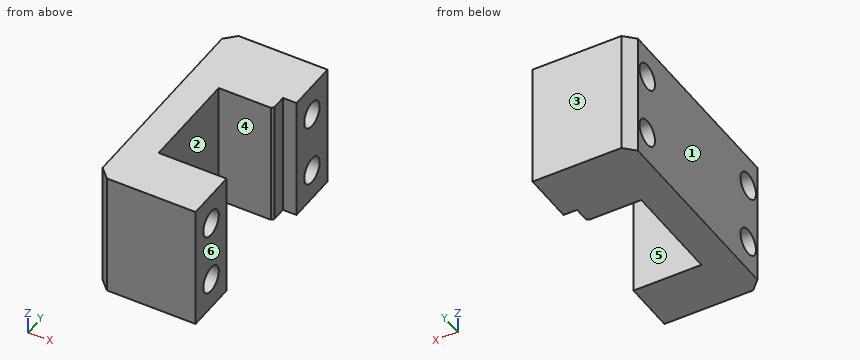
from build123d import *

# Parameters (mm, degrees)
EXTRUDE_1_DEPTH    = 12
CHAMFER_1_SIZE     = 0.2
HOLE_WIZARD_M3_2_D = 2.5
CHAMFER_2_SIZE     = 1


with BuildPart() as part:
    # 草图1 → 凸台-拉伸1 (new body)
    with BuildSketch(Plane.XY):
        Polygon((0, 0), (0, 21.31), (9.5, 21.31), (9.5, 16.31), (8.2, 16.31), (8.2, 14.71), (3, 14.71), (3, 5), (9.5, 5), (9.5, 0), align=None)
    extrude(amount=EXTRUDE_1_DEPTH)

    # 倒角1
    chamfer_1_edges = [part.edges().sort_by_distance(p)[0] for p in [
        (8.2, 14.71, 6),
    ]]
    chamfer(chamfer_1_edges, length=CHAMFER_1_SIZE)

    # M3 螺纹孔2 (through all)
    with Locations(Plane(origin=(0, 2.5, 3), x_dir=(0, 0, -1), z_dir=(-1, 0, 0))):
        with Locations((0, 0), (-6, 0), (-6, -16.31), (0, -16.31)):
            Hole(HOLE_WIZARD_M3_2_D / 2)

    # 倒角2
    chamfer_2_edges = [part.edges().sort_by_distance(p)[0] for p in [
        (0, 0, 6),
        (0, 21.31, 6),
    ]]
    chamfer(chamfer_2_edges, length=CHAMFER_2_SIZE)


solid = part.part
Can you work these out from the model? Positions are in its coordinate system, mm. Face numbers are marked on the shaded views. A direction names the side the tool comes from. Coordinates: 2 decimals unless noted, no trailing zeros. Write each loop counter-clockwise with the first axis right and the second up, starting at its lowest first coordinate (ties: lowest second). Pieces come first, ordered by that corner, then holes. Notation, with made-up numbers: (-20, 22) -> (27, 22) arc R24 ccw to (27, 58) -> close; hole circle Ø3 at (77, 70). An arc over 180 degrees is marked (long way). Write each question's results on one line, items separated by ' | '. Start each with the question number.
Q1. I'm going to push flat-ended pins straight in: pin 1 (4 mm diameter, centred on x = 4.5, y = 2.5, fed in from -Z); pin 2 (0.7 mm diameter, centred on y = 15.5, z = 5, fed in from +X); pin 3 (2 mm diameter, centred on y = 18.81, z = 9, fed in from -X) (3 decimals). Where does each tip first touch, or does it pass through?
Q2. Imagine slicing it at A-A (y = 2.5). Write out the boundary of the cut face in (x, z), then the cut area to 3 significant figures.
Q3. Imagine slicing it at D-D (x = 2). Write out the boundary of the cut face in (y, z).
Q4. We'd pull the mould along Y, two halves only. Please class the marked faces 1, 2, 3 and 4: +Y half, -Y half, draft (parallel to the pull), parting line (faces both ways), or undercut.
Q5. Imagine slicing it at C-C (x = 5.5). Write out the boundary of the cut face in (y, z).
Q6. On a 3-axis mill with a long thin cutter (end or side, diameter ignored), from which of +Z, -Z, +X, -X, +Y, -Y can I reach the whole of each face in a straight line? I mean the marked faces 5 and 6. Say none if no direction works.
Q7. Imagine slicing it at B-B (z = 4). Write out the boundary of the cut face in (x, y), then the cut area to 3 significant figures.
Q8. If I drill on probe 1 along Y at (x, z) = (6.75, 9); probe 2 along Z at (x, y) = (4.5, 18.81); probe 3 along Y at (x, z) = (2.75, 9), over which ranges is the centre line in solid material (lowest first)?
Taken from the geometry:
1) pin 1: stops at z = 0 | pin 2: stops at x = 8.2 | pin 3: passes through
2) outline: (0, 0) -> (9.5, 0) -> (9.5, 1.75) -> (0, 1.75) -> close; (0, 4.25) -> (9.5, 4.25) -> (9.5, 7.75) -> (0, 7.75) -> close; (0, 10.25) -> (9.5, 10.25) -> (9.5, 12) -> (0, 12) -> close | area: 66.5 mm^2
3) outline: (0, 0) -> (21.31, 0) -> (21.31, 12) -> (0, 12) -> close; hole circle Ø2.5 at (2.5, 3); hole circle Ø2.5 at (2.5, 9); hole circle Ø2.5 at (18.81, 3); hole circle Ø2.5 at (18.81, 9)
4) face 1: draft | face 2: undercut | face 3: +Y half | face 4: undercut
5) outline: (0, 0) -> (5, 0) -> (5, 12) -> (0, 12) -> close; (14.71, 0) -> (21.31, 0) -> (21.31, 12) -> (14.71, 12) -> close; hole circle Ø2.5 at (2.5, 3); hole circle Ø2.5 at (2.5, 9); hole circle Ø2.5 at (18.81, 3); hole circle Ø2.5 at (18.81, 9)
6) face 5: +Z, -Z, +X | face 6: +Z, -Z, +X, +Y, -Y
7) outline: (0, 1) -> (1, 0) -> (9.5, 0) -> (9.5, 1.75) -> (0, 1.75) -> close; (0, 3.25) -> (9.5, 3.25) -> (9.5, 5) -> (3, 5) -> (3, 14.71) -> (8, 14.71) -> (8.2, 14.91) -> (8.2, 16.31) -> (9.5, 16.31) -> (9.5, 18.06) -> (0, 18.06) -> close; (0, 19.56) -> (9.5, 19.56) -> (9.5, 21.31) -> (1, 21.31) -> (0, 20.31) -> close | area: 108 mm^2
8) probe 1: y = 0 to 1.25, 3.75 to 5, 14.71 to 17.56, 20.06 to 21.31 | probe 2: z = 0 to 1.75, 4.25 to 7.75, 10.25 to 12 | probe 3: y = 0 to 1.25, 3.75 to 17.56, 20.06 to 21.31
